Design review of the part shown in the three views and the two pictorial views. Dimensions are in mm from the part's minimum x, y and z. Coordinates: 2 decimals unless noted, no trailing zeros. Answer in a Markdown table with one row per item. Add a question column.
Item 1: Clearance check with flat-ended pins moving along their axes: P1, Ø2, axis at y = 1, z = 75, coming from the -X side; P2, Ø2, axis at y = 1, z = 48.5, coming from the -X side; P3, Ø2.5, axis at x = 3.5, y = 3.5, coming from the -Z side. State where each tip first meets the part, or that it passes through.
Item 2: Take a section at A-A, the plane y = 2.7. Give the number of separate pieces and of enclosed holes in the cut face, and give its area (3 significant figures).
Item 3: To check wall thickness, follow line 1 (Z direction, x = 238.75, y = 3.4); line 2 (X direction, y = 3.1, z = 148.5); line 3 (Z direction, x = 20, y = 3.75). State the ranges of each line that lie inside material, in increasing order.
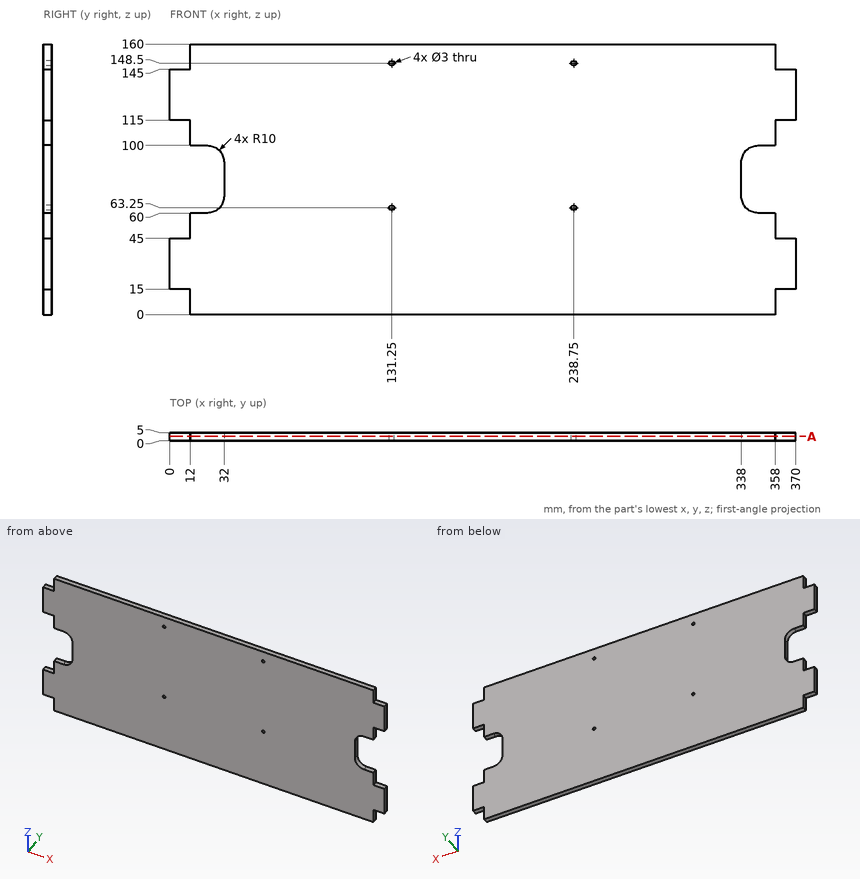
Answers:
| question | item | result |
|---|---|---|
| 1 | P1 | stops at x = 32 |
| 1 | P2 | stops at x = 12 |
| 1 | P3 | stops at z = 15 |
| 2 | separate pieces | 1 |
| 2 | enclosed holes | 4 |
| 2 | area | 55,300 mm^2 |
| 3 | line 1 | z = 0 to 61.75, 64.75 to 147, 150 to 160 |
| 3 | line 2 | x = 12 to 129.75, 132.75 to 237.25, 240.25 to 358 |
| 3 | line 3 | z = 0 to 60, 100 to 160 |
